Job drawing, mm, ordinate dimensions from the low corner. One solid piece. Give positions to 0.01 mm unless a question says otherwise; leave off trailing zeros. Order: outer loops, then holes, each group sorted by start corner. A loop starts at its lowest first (then second) coordinate and runs counter-clockwise, first axis right, second up.
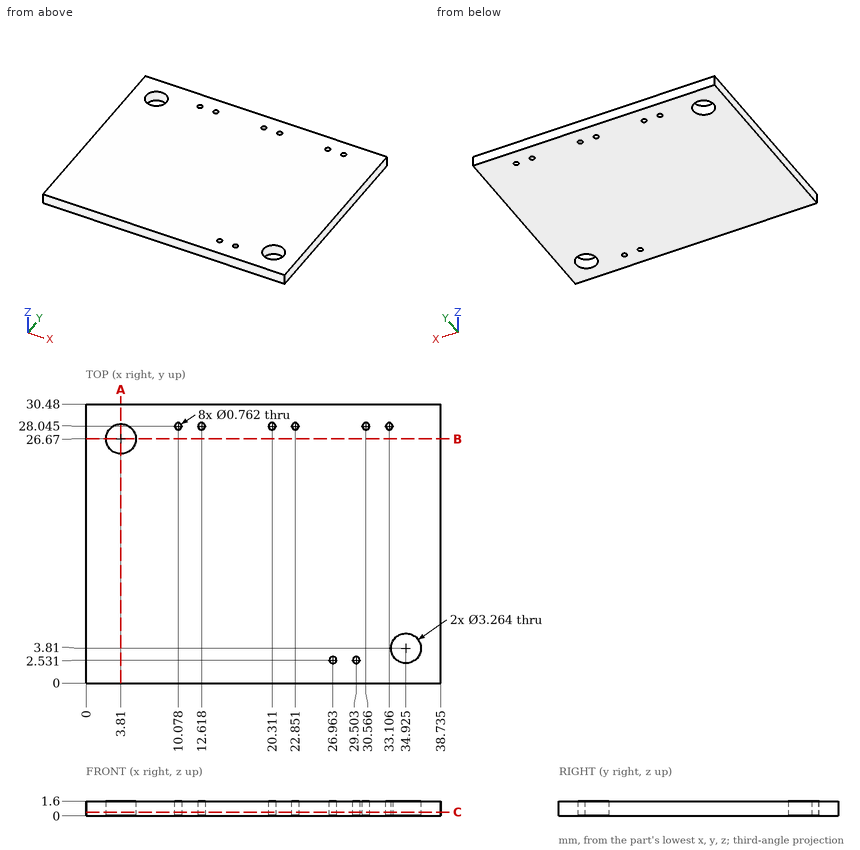
Item 1: Band-saw the part on A-A on x = 3.81. List the corners of the cut face in (y, z).
Item 2: Drill centre lines: probe 1 along Y at (x, z) = (29.5, 0.65); probe 2 along X at (y, z) = (5, 0.6) (1 decimal); probe 3 along Y at (x, z) = (33, 0.9). Where is each one in solid material? Low to high.
Item 3: Band-saw the part on C-C on z = 0.4. Give the number of separate pieces and of enclosed holes in the cut face, plus the area to 3 significant figures.
Item 4: Band-saw the part on B-B on y = 26.67. List the corners of the cut face in (x, z) (1 decimal).
Item 5: Drop a flat-ended pin along its axis: P1, Ø2, axis at x = 3.81, y = 26.67, coming from the +Z side. Give the stop position or say it passes through.
Working result:
1. outline: (0, 0) - (25.04, 0) - (25.04, 1.6) - (0, 1.6) - close; (28.3, 0) - (30.48, 0) - (30.48, 1.6) - (28.3, 1.6) - close
2. probe 1: y = 0 to 2.15, 2.91 to 30.48
2. probe 2: x = 0 to 33.8, 36 to 38.7
2. probe 3: y = 0 to 27.68, 28.41 to 30.48
3. separate pieces: 1
3. enclosed holes: 10
3. area: 1,160 mm2
4. outline: (0, 0) - (2.2, 0) - (2.2, 1.6) - (0, 1.6) - close; (5.4, 0) - (38.7, 0) - (38.7, 1.6) - (5.4, 1.6) - close
5. P1: passes through
